from build123d import *

# Parameters (mm, degrees)
F1_DEPTH = 2.38125
F4_R     = 3.96875
F5_DEPTH = 25.4
F7_DEPTH = 25.4


with BuildPart() as f1:
    # F0 (on Front) → F1 (new body)
    with BuildSketch(Plane.XZ):
        with BuildLine():
            Line((60.325, 19.05), (7.9375, 19.05))
            ThreePointArc((7.9375, 19.05), (2.32484, 16.72516), (0, 11.1125))
            Line((0, 11.1125), (0, 0))
            Line((0, 0), (9.525, 0))
            Line((9.525, 0), (13.483182, 9.525))
            ThreePointArc((13.483182, 9.525), (14.624025, 10.091332), (15.875, 10.330743))
            Line((15.875, 10.330743), (60.325, 12.7))
            Line((60.325, 12.7), (60.325, 19.05))
        make_face()
    extrude(amount=F1_DEPTH)

    # F4 (on face) → F5 (cut)
    with BuildSketch(Plane.XZ.offset(2.38125)):
        with Locations((7.9375, 11.1125)):
            Circle(F4_R)
    extrude(amount=-F5_DEPTH, mode=Mode.SUBTRACT)

    # F6 (on face) → F7 (cut)
    with BuildSketch(Plane.XY.offset(19.05)):
        Polygon((60.325, 0), (45.2374, 0), (60.325, -0.819355), align=None)
        Polygon((60.325, -2.38125), (60.325, -1.561895), (45.2374, -2.38125), align=None)
    extrude(amount=-F7_DEPTH, mode=Mode.SUBTRACT)


solid = f1.part
CAD build for the part. Positions are in the model's coordinates, mm. Coordinates: 2 decimals unless noted, no trailing zeros. Order: outer loops, then holes, each group sorted by start corner. A loop starts at its lowest first (then second) coordinate and runs counter-clockwise, first axis right, second up.
Item 1: Band-saw the part on A-A on z = 14.5. List the corners of the cut face in (x, y) (3 decimals), plus the area to 3 significant figures.
Check sheet entries:
outline: (0.759, -2.381) - (5.87, -2.381) - (5.87, 0) - (0.759, 0) - close; (10.005, -2.381) - (45.237, -2.381) - (60.325, -1.562) - (60.325, -0.819) - (45.237, 0) - (10.005, 0) - close
area: 120 mm2
Item 2: Two-plate mould, pull along X, no slides. Class faces 1 (the face through (34, -1, 19.05)), 2 (the face through (2.4, -1.2, 16.8)), 3 (the face through (4.788, -1.207, 8.698)): +X half, -X half, draft (parallel to the pull), parting line (faces both ways), or undercut.
Check sheet entries:
face 1: draft
face 2: -X half
face 3: undercut
Item 3: Band-saw the part on C-C on x = 43. List the corners of the cut face in (y, z), plus the area to 3 significant figures.
Check sheet entries:
outline: (-2.38, 11.78) - (0, 11.78) - (0, 19.05) - (-2.38, 19.05) - close
area: 17.3 mm2
Item 4: Band-saw the part on D-D on z = 1.5. List the corners of the cut face in (x, y).
Check sheet entries:
outline: (0, -2.38) - (10.15, -2.38) - (10.15, 0) - (0, 0) - close
Item 5: Drill centre lines: L1, parallel to Z at x = 5.5, y = -0.9; L2, parallel to Z at x = 9.5, y = -1.5; L3, parallel to X at y = -1.25, z = 14 (3 decimals). Where is each one in solid material? Low to high.
Check sheet entries:
L1: z = 0 to 7.98, 14.24 to 18.67
L2: z = 0 to 7.46, 14.76 to 19.05
L3: x = 0.544 to 5.215, 10.66 to 60.325
